Input: part model. Units: mm. Frame: model coordinates. Face numbers are marked on the shaded views. A direction names the side the tool comes from. Coordinates: 2 decimals unless noted, no trailing zeros. Loops run counter-clockwise (first coordinate to the right, second up) from the corner with the lowest first, then second, coordinate; pieces in that order, holes last. Notation, with made-up numbers: (-31, 40) -> (17, 40) arc R17 cw to (17, 64) -> close; hole circle Ø3 at (78.5, -34). An arc over 180 degrees is marked (long way). Answer as a JSON object with one key per item and string values.
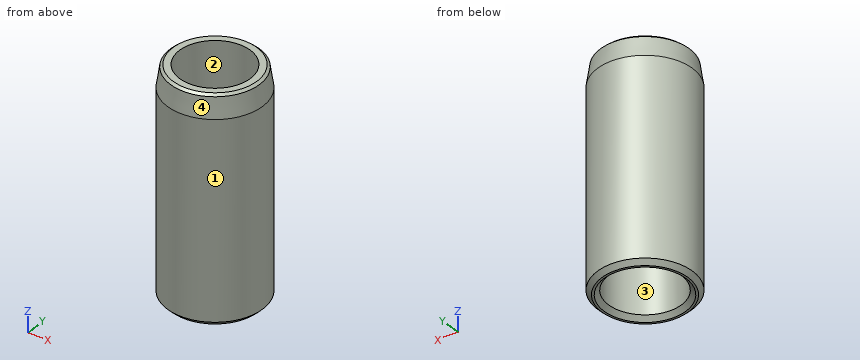
Autodesk Inventor part; units mm, degrees
ref_plane "Plan de construction2" through (14, 0, 0) normal (1, 0, 0) x (0, 1, 0)
ref_plane "XZ Plane" through (0, 0, 0) normal (0, 1, 0) x (-1, 0, 0)
ref_plane "XY Plane" through (0, 0, 0) normal (0, 0, 1) x (1, 0, 0)
sketch "Esquisse1" plane through (0, 0, 0) normal (1, 0, 0) x (0, 1, 0)
  line L0 (0, 0) -> (0, 17.1522)
  line L1 (8, 50) -> (8, 36)
  line L2 (8, 36) -> (6, 36)
  line L3 (6, 36) -> (6, 30)
  line L4 (6, 30) -> (8.25, 23.8182)
  line L5 (8.25, 23.8182) -> (8.25, 1)
  line L6 (8.25, 1) -> (9.25, 0)
  line L7 (9.25, 0) -> (9.75, 0)
  line L8 (8, 50) -> (10, 50)
  line L9 (10, 50) -> (10.75, 45)
  line L10 (10.75, 45) -> (10.75, 1)
  line L11 (10.75, 1) -> (9.75, 0)
  dimension "d0" = 160
  dimension "d1" = 6
  dimension "d2" = 14
  dimension "d4" = 16
  dimension "d6" = 16.5
  dimension "d8" = 1
  dimension "d9" = 1
  dimension "d10" = 30
  dimension "d11" = 2
  dimension "d12" = 2
  dimension "d13" = 21.5
  dimension "d14" = 2.5
  dimension "d15" = 5
  dimension "d19" = 1
  dimension "d20" = 1
  dimension "d48" = 2.75
  dimension "d49" = 4.75
revolve "Révolution1" add sketch "Esquisse1" angle 360 about axis through (0, 0, 0) along (0, 0, 1)
thread "Filetage1"
ref_plane "Plan de construction2" through (14, 0, 0) normal (1, 0, 0) x (0, 1, 0)
chamfer "Chanfrein4" distance 0.5 angle 45 1 edges at (0, -10, 50)
properties part number "support_douille" material "Aluminium 6061"
1. Access query for the marked faces 1 and 2. Directions: +Z, -Z, +X, -X, +Y, -Y. A direction counts if a zero-diameter tool reaches every point of the face in a straight line with its end or side. Return the directions, or none.
Reply:
{"face 1": "+Z, -Z", "face 2": "+Z"}
2. Section query A-A (y = 0). Return loops of the section in (x, z).
Reply:
{"outline": "(-10.75, 1) -> (-9.75, 0) -> (-9.25, 0) -> (-8.25, 1) -> (-8.25, 23.82) -> (-6, 30) -> (-6, 36) -> (-8, 36) -> (-8, 50) -> (-9.5, 50) -> (-10.07, 49.51) -> (-10.75, 45) -> close; (6, 30) -> (8.25, 23.82) -> (8.25, 1) -> (9.25, 0) -> (9.75, 0) -> (10.75, 1) -> (10.75, 45) -> (10.07, 49.51) -> (9.5, 50) -> (8, 50) -> (8, 36) -> (6, 36) -> close"}
3. Section query C-C (z = 28.5). Return loops of the section in (x, y).
Reply:
{"outline": "circle Ø21.5 at (0, 0); hole circle Ø13.09 at (0, 0)"}
4. Pin query (flat end, axial travel): P1, Ø8, axis at x = 1, y = 0, coming from the +Z side; P2, Ø1, axis at x = -4.5, y = -6.5, coming from the -Z side; P3, Ø10, axis at y = -8, z = 25.5, coming from the +X side; P4, Ø4, axis at y = 2.5, z = 31, coming from the +X side. Return the tip coordinate at first contact, or that it passes through.
Reply:
{"P1": "passes through", "P2": "stops at z = 0.84", "P3": "stops at x = 10.32", "P4": "stops at x = 10.74"}
5. Mould query, pull axis Y, two halves, no side actions, for the marked faces 3 and 4. Classes: pulls with the +Y half, pulls with the -Y half, needs draft (parallel to the pull), parting line crosses it, or undercut.
Reply:
{"face 3": "undercut", "face 4": "parting line crosses it"}
6. Section query B-B (z = 6.5). Return loops of the section in (x, y), plus the area to 3 significant figures.
Reply:
{"outline": "circle Ø21.5 at (0, 0); hole circle Ø16.5 at (0, 0)", "area": "149 mm2"}
7. Line query: line 1 along Y through (x, z) = (0, 40.5); line 2 along Y through (x, z) = (0, 34.4); line 3 along X through (y, z) = (0, 7.25). Output: solid intervals per line, ascending.
Reply:
{"line 1": "y = -10.75 to -8, 8 to 10.75", "line 2": "y = -10.75 to -6, 6 to 10.75", "line 3": "x = -10.75 to -8.25, 8.25 to 10.75"}
